Autodesk Inventor part; units mm, degrees
ref_plane "YZ Plane" through (0, 0, 0) normal (1, 0, 0) x (0, 1, 0)
ref_plane "XZ Plane" through (0, 0, 0) normal (0, 1, 0) x (-1, 0, 0)
ref_plane "XY Plane" through (0, 0, 0) normal (0, 0, 1) x (1, 0, 0)
sketch "Boceto1" plane through (0, 0, 0) normal (0, 0, 1) x (1, 0, 0)
  circle A0 centre (-11.375, 0) radius 0.975
  arc A1 (13.3142, 0.145) -> (12.3392, 1.12) centre (12.3392, 0.145) ccw
  line L0 (12.3392, 1.12) -> (9.6855, 1.12)
  line L1 (18.4935, 0) -> (-19.3273, 0)
  arc A2 (12.3392, -1.12) -> (13.3142, -0.145) centre (12.3392, -0.145) ccw
  line L2 (12.3392, -1.12) -> (9.6855, -1.12)
  line L3 (0, 0) -> (0, 1.0605)
  arc A3 (-12.3392, 1.12) -> (-13.3142, 0.145) centre (-12.3392, 0.145) ccw
  line L4 (-12.3392, 1.12) -> (-9.6855, 1.12)
  line L5 (-12.3392, -1.12) -> (-9.6855, -1.12)
  arc A4 (-13.3142, -0.145) -> (-12.3392, -1.12) centre (-12.3392, -0.145) ccw
  line L6 (-5.1219, 12.666) -> (5.1219, 12.666)
  arc A5 (-5.1219, 8.2963) -> (-9.6855, 1.12) centre (0, 0) ccw
  arc A6 (-9.6855, -1.12) -> (9.6855, -1.12) centre (0, 0) ccw
  arc A7 (9.6855, 1.12) -> (5.1219, 8.2963) centre (0, 0) ccw
  line L7 (-5.1219, 12.666) -> (-5.1219, 8.2963)
  line L8 (5.1219, 12.666) -> (5.1219, 8.2963)
  line L9 (-13.3142, 0.145) -> (-13.3142, -0.145)
  line L10 (13.3142, 0.145) -> (13.3142, -0.145)
  circle A8 centre (11.375, 0) radius 0.975
  point P0 (13.3033, 0)
  point P1 (13.3142, 0)
  point P2 (5.1219, 10.4811)
  dimension "d2" = 1.95
  dimension "d4" = 11.375
  dimension "d7" = 1.95
  dimension "d12" = 2.6537
  dimension "d20" = 9.75
  dimension "d21" = 2.24
  dimension "d22" = 12.666
  dimension "d24" = 10.2439
  dimension "d25" = 10.2439
  dimension "d26" = 4.3697
  dimension "d29" = 1.95
  dimension "d30" = 11.375
extrude "Extrusión3" add sketch "Boceto1" along normal blind 0.5 contours L1 A8 L10 A2 L2 A6 L5 A4 L9 A0 | A0 L1 L9 A3 L4 A5 L7 L6 L8 A7 L0 A1 L10 A8
sketch "Boceto2" plane through (0, 0, 0) normal (0, 0, -1) x (-1, 0, 0)
  line L0 (-5.1219, 12.666) -> (5.1219, 12.666)
  line L1 (-5.1219, 8.2963) -> (-5.1219, 12.666)
  arc A0 (-5.1219, 8.2963) -> (-9.6855, 1.12) centre (0, 0) ccw
  line L2 (-12.3392, 1.12) -> (-9.6855, 1.12)
  arc A1 (-12.3392, 1.12) -> (-13.3142, 0.145) centre (-12.3392, 0.145) ccw
  line L3 (-13.3142, -0.145) -> (-13.3142, 0.145)
  arc A2 (-13.3142, -0.145) -> (-12.3392, -1.12) centre (-12.3392, -0.145) ccw
  line L4 (-9.6855, -1.12) -> (-12.3392, -1.12)
  arc A3 (-9.6855, -1.12) -> (9.6855, -1.12) centre (0, 0) ccw
  line L5 (12.3392, -1.12) -> (9.6855, -1.12)
  arc A4 (12.3392, -1.12) -> (13.3142, -0.145) centre (12.3392, -0.145) ccw
  line L6 (13.3142, 0.145) -> (13.3142, -0.145)
  arc A5 (13.3142, 0.145) -> (12.3392, 1.12) centre (12.3392, 0.145) ccw
  line L7 (9.6855, 1.12) -> (12.3392, 1.12)
  arc A6 (9.6855, 1.12) -> (5.1219, 8.2963) centre (0, 0) ccw
  line L8 (5.1219, 12.666) -> (5.1219, 8.2963)
  arc A7 (-5.1219, 8.2963) -> (5.1219, 8.2963) centre (0, 0) ccw
  line L9 (-5.1219, 8.2963) -> (-5.1219, 12.666)
  line L10 (-5.1219, 8.2963) -> (-5.1219, 12.666)
  line L11 (-5.1219, 12.666) -> (5.1219, 12.666)
  line L12 (5.1219, 8.2963) -> (5.1219, 12.666)
  point P0 (9.6855, -1.12)
  point P1 (-9.6855, 1.12)
extrude "Extrusión4" add sketch "Boceto2" along normal blind 10 contours L0 L8 A6 A7 A3 A0 L1
sketch "Boceto3" plane through (0, 0, 0) normal (0, 0, -1) x (-1, 0, 0)
  arc A0 (-5.1219, 8.2963) -> (5.1219, 8.2963) centre (0, 0) ccw
  line L0 (5.6225, 13.166) -> (-5.6225, 13.166)
  arc A1 (5.6225, 7.9656) -> (-5.6225, 7.9656) centre (0, 0) ccw
  line L1 (5.1219, 12.666) -> (-5.1219, 12.666)
  line L2 (5.6225, 13.166) -> (5.6225, 7.9656)
  line L3 (-5.6225, 13.166) -> (-5.6225, 7.9656)
  point P0 (0, 13.166)
  point P1 (0, 12.666)
  point P2 (-5.6225, 7.9656)
  point P3 (-5.1219, 8.2963)
  point P4 (5.1219, 8.2963)
  point P5 (5.6225, 7.9656)
  dimension "d38" = 11.245
  dimension "d39" = 13.166
extrude "Extrusión6" add sketch "Boceto3" along normal blind 10 contours A0 L3 L0 L2 A1
sketch "Boceto4" plane through (0, 0, 0.5) normal (0, 0, 1) x (1, 0, 0)
  circle A0 centre (0, -4.8124) radius 2.25
  point P0 (0, 0)
  dimension "d42" = 4.5
extrude "Extrusión7" add sketch "Boceto4" along normal blind 1
sketch "Boceto5" plane through (0, -4.8124, 1.5) normal (0, 0, 1) x (1, 0, 0)
  circle A0 centre (0, 0) radius 1
  point P0 (0, 4.8124)
  dimension "d45" = 2
extrude "Extrusión8" add sketch "Boceto5" along normal blind 3
properties part number "stepper_motor" material "Acero, suave"
Part model, mm, in its own coordinate system. A direction names the side the tool comes from. Round coordinates to 2 decimals unless told otherwise and drop trailing zeros. Write each loop counter-clockwise with the first axis right and the second up, starting at its lowest first coordinate (ties: lowest second). Pieces come first, ordered by that corner, then holes. Notation, with made-up numbers: M -7.5,-28 L 18.5,-28 A19 ccw 18.5,-15 Z; hole C 48.25,-3.5 d5. An arc over 180 degrees is marked long. Return JSON: item names as keys, results as strings. Group by question number.
(1) Saw through at C-C on y = 6.5. Write the cut outline in (x, z).
(2) Pin check, flat tips, straight feed: pin 1 Ø1.8 at (x, y) = (-11, 0) entering from -Z; pin 2 Ø5 at (x, y) = (8, -3.5) entering from +Z; pin 3 Ø2 at (y, z) = (-2, 2) entering from +X. Stop position of each tip, or through.
(3) Two-plate mould, pull along X, no slides. Class faces 4 (the face through (0, -5, 4.5)), 5 (the face through (10.4, 0, 0.2)), 6 (the face through (-0.13, -5.804, 2.979)): +X half, -X half, draft (parallel to the pull), parting line (faces both ways), or undercut.
(4) Saw through at A-A on x = -10.75. Write the cut outline in (y, z).
(5) Saw through at B-B on z = -3.25. Write the cut outline in (x, y).
(6) Saw through at D-D on x = 0. Write the cut outline in (y, z).
(7) Which spindle directions (+Z, -Z, +X, -X, +Y, -Y) get a long thin tool onto all of the face, cutting with end or side? Do faces 1 (the face through (-5.622, 11, -5)), 2 (the face through (0, -6, 1.5)), 3 (the face through (5.622, 11, -5)). Say none if no direction does.
(8) Drill centre lines: probe 1 along X at (y, z) = (0, 0.3); probe 2 along Z at (x, y) = (0, 8.5); probe 3 along Z at (x, y) = (-10, -0.5). Where is each one in solid material? Low to high.
Returned:
{
 "1": {"outline": "M -7.27,-10 L 7.27,-10 L 7.27,0.5 L -7.27,0.5 Z"},
 "2": {"pin 1": "z = 0", "pin 2": "z = 0.5", "pin 3": "x = 1.13"},
 "3": {"face 4": "draft", "face 5": "undercut", "face 6": "parting line"},
 "4": {"outline": "M -1.12,0 L -0.75,0 L -0.75,0.5 L -1.12,0.5 Z; M 0.75,0 L 1.12,0 L 1.12,0.5 L 0.75,0.5 Z"},
 "5": {"outline": "M -9.69,-1.12 A9.75 ccw 9.69,-1.12 A9.75 ccw 9.69,1.12 A9.75 ccw 5.62,7.97 L 5.62,13.17 L -5.62,13.17 L -5.62,7.97 A9.75 ccw -9.69,1.12 A9.75 ccw Z"},
 "6": {"outline": "M -9.75,-10 L 13.17,-10 L 13.17,0 L 12.67,0 L 12.67,0.5 L -2.56,0.5 L -2.56,1.5 L -3.81,1.5 L -3.81,4.5 L -5.81,4.5 L -5.81,1.5 L -7.06,1.5 L -7.06,0.5 L -9.75,0.5 Z"},
 "7": {"face 1": "+Z, -Z, -X, +Y", "face 2": "+Z", "face 3": "+Z, -Z, +X, +Y"},
 "8": {"probe 1": "-13.31 to -12.35, -10.4 to 10.4, 12.35 to 13.31", "probe 2": "-10 to 0.5", "probe 3": "0 to 0.5"}
}
